Read the model definition and answer for the solid it produces. Units are mm, in the model's axes. Face numbers are marked on the shaded views. Coordinates: 2 decimals unless noted, no trailing zeros. Order: outer loops, then holes, each group sorted by start corner. A loop starts at its lowest first (then second) coordinate and runs counter-clockwise, first axis right, second up. Notation, with made-up numbers: (53, -6.75) - (103, -6.75) arc R15 cw to (103, 15.25) - close; hole circle Ø8 at (14.25, -21). An arc over 180 degrees is marked (long way). Write item = value, one per line.
from build123d import *

# Parameters (mm, degrees)
SKETCH1_R      = 0.762
EXTRUDE1_DEPTH = 10.414
SKETCH2_R      = 0.889
EXTRUDE2_DEPTH = 0.127
EXTRUDE3_START = 0.127
SKETCH3_R      = 0.889
EXTRUDE3_DEPTH = 0.127
FILLET1_R      = 0.2032


with BuildPart() as part:
    # Sketch1 → Extrude1 (new body)
    with BuildSketch(Plane(origin=(0, 0, 0), x_dir=(0, 0, -1), z_dir=(1, 0, 0))):
        Circle(SKETCH1_R)
    extrude(amount=EXTRUDE1_DEPTH)

    # Sketch2 → Extrude2 (add)
    with BuildSketch(Plane(origin=(10.414, 0, 0), x_dir=(0, 0, -1), z_dir=(1, 0, 0))):
        Circle(SKETCH2_R)
    extrude(amount=EXTRUDE2_DEPTH)

    # Sketch3 → Extrude3 (add)
    with BuildSketch(Plane.ZY.offset(EXTRUDE3_START)):
        with Locations(Location((0, 0, 0), (0, 0, 180))):
            Circle(SKETCH3_R)
    extrude(amount=-EXTRUDE3_DEPTH)

    # Fillet1
    # the kernel refuses this fillet: 0.2032 mm, written as the material it takes off along each edge
    with BuildSketch(Plane(origin=(10.541, 0, 0), x_dir=(0, 0, -1), z_dir=(0, -1, 0))) as fillet1_piece_1:
        with BuildLine():
            CenterArc((0.700628558, -0.2032), FILLET1_R, 22.024312837, 67.975687163)
            Line((0.700628558, 0), (0.700628558, 0.004064))
            Line((0.700628558, 0.004064), (0.889, 0.004064))
            Line((0.889, 0.004064), (0.893064, 0))
            ThreePointArc((0.893064, 0), (0.893064, -0.0635), (0.892767429, -0.125476))
            Line((0.892767429, -0.125476), (0.889, -0.127))
        make_face()
    revolve(axis=Axis((10.541, 0, 0), (1, 0, 0)), mode=Mode.SUBTRACT)
    with BuildSketch(Plane(origin=(-0.127, 0, 0), x_dir=(0, 0, -1), z_dir=(0, 1, 0))) as fillet1_piece_2:
        with BuildLine():
            CenterArc((0.700628558, -0.2032), FILLET1_R, 22.024312837, 67.975687163)
            Line((0.700628558, 0), (0.700628558, 0.004064))
            Line((0.700628558, 0.004064), (0.889, 0.004064))
            Line((0.889, 0.004064), (0.893064, 0))
            ThreePointArc((0.893064, 0), (0.893064, -0.0635), (0.892767429, -0.125476))
            Line((0.892767429, -0.125476), (0.889, -0.127))
        make_face()
    revolve(axis=Axis((-0.127, 0, 0), (-1, 0, 0)), mode=Mode.SUBTRACT)


solid = part.part
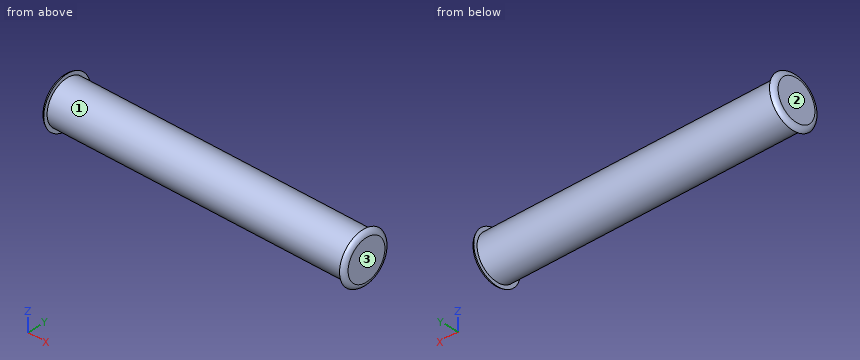
1) A flat-ended cylindrical pin translates along its axis: pin 1 Ø1 at (x, y) = (8.5, -0.5) entering from +Z. Find the tip coordinate at first contact, or state that the pin passes through.
Returned:
pin_1 = 0.76
2) The part is cut by section C-C (x = 2.5). Determine the outline of the cut face in (y, z).
Returned:
outline = circle Ø1.52 at (0, 0)
3) The part is cut by section A-A (z = 0). Determine the outline of the cut face in (x, y), and give its area (3 significant figures).
Returned:
outline = (-0.13, -0.7) arc R0.2 ccw to (0, -0.89) - (0, -0.76) - (10.41, -0.76) - (10.41, -0.89) arc R0.2 ccw to (10.54, -0.7) - (10.54, 0.7) arc R0.2 ccw to (10.41, 0.89) - (10.41, 0.76) - (0, 0.76) - (0, 0.89) arc R0.2 ccw to (-0.13, 0.7) - close
area = 16.3 mm^2
4) Determine the mould class of the marked faces 1, 2 and 3 for opening direction X: pulls with the +X half, pulls with the -X half, needs draft (parallel to the pull), parting line crosses it, or undercut.
Returned:
face_1 = undercut
face_2 = pulls with the -X half
face_3 = pulls with the +X half
5) Straight lines are drawn through the part: line 1 along Z through (x, y) = (2.25, 0.3); line 2 along Y through (x, z) = (10.25, 0). For each, find the intervals that lie inside material, in ascending order. Write a range as from..to.
Returned:
line_1 = -0.7..0.7
line_2 = -0.76..0.76
